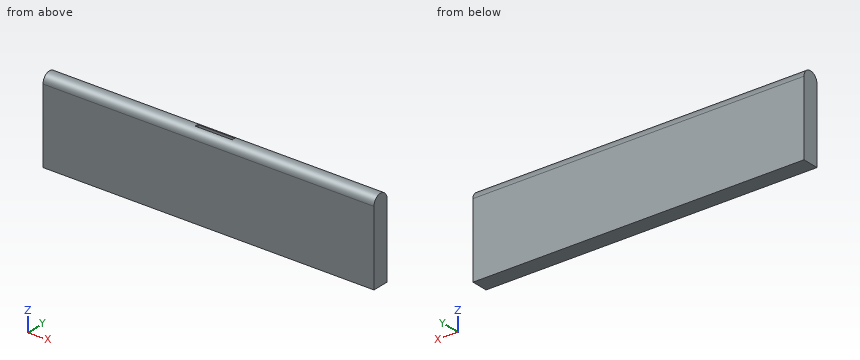
Autodesk Inventor part; units mm, degrees
ref_plane "YZ Plane" through (0, 0, 0) normal (1, 0, 0) x (0, 1, 0)
ref_plane "XZ Plane" through (0, 0, 0) normal (0, 1, 0) x (-1, 0, 0)
ref_plane "XY Plane" through (0, 0, 0) normal (0, 0, 1) x (1, 0, 0)
sketch "Sketch2" plane through (0, 0, 0) normal (0, 1, 0) x (-1, 0, 0)
  line L0 (0, 0) -> (-100, 0)
  line L1 (-100, 0) -> (-100, 25)
  line L2 (-100, 25) -> (0, 25)
  line L3 (0, 25) -> (0, 0)
  dimension "d10" = 100
  dimension "d11" = 25
extrude "Extrusion2" add sketch "Sketch2" along normal blind 5
sketch "Sketch3" plane through (0, 0, 25) normal (0, 0, 1) x (1, 0, 0)
  line L0 (0, 0) -> (100, 0) construction
  line L1 (0, 0) -> (44.4, 0) construction
  line L2 (44.4, 0) -> (44.4, 2) construction
  line L3 (44.4, 2) -> (0, 2) construction
  line L4 (0, 2) -> (0, 0) construction
  line L5 (44.4, 2) -> (55.6, 2)
  line L6 (55.6, 2) -> (55.6, 3)
  line L7 (55.6, 3) -> (44.4, 3)
  line L8 (44.4, 3) -> (44.4, 2)
  dimension "d14" = 44.4
  dimension "d15" = 2
  dimension "d16" = 11.2
  dimension "d17" = 1
extrude "Extrusion3" cut sketch "Sketch3" against normal blind 12.5
fillet "Fillet2" radius 2.5 2 edges at (50, 5, 25) (50, 0, 25)
shell "Shell1" thickness 1 removed faces 0
properties part number "RCPlaneElevator"
CAD build for the part. Positions are in the model's coordinates, mm. Coordinates: 2 decimals unless noted, no trailing zeros. Loops run counter-clockwise (first coordinate to the right, second up) from the corner with the lowest first, then second, coordinate; pieces in that order, holes last. Notation, with made-up numbers: (39.25, -30.75) - (89.25, -30.75) arc R25 cw to (89.25, -7.75) - close; hole circle Ø2 at (47.5, 56.25). An arc over 180 degrees is marked (long way). Return JSON: item names as keys, results as strings.
1. Band-saw the part on C-C (z = 19.5). Give the cut face in (x, y).
Result:
{"outline": "(0, 0) - (100, 0) - (100, 5) - (0, 5) - close; hole (1, 1) - (43.4, 1) - (43.4, 4) - (1, 4) - close; hole (44.4, 2) - (55.6, 2) - (55.6, 3) - (44.4, 3) - close; hole (56.6, 1) - (99, 1) - (99, 4) - (56.6, 4) - close"}
2. Band-saw the part on A-A (z = 2.75). Give the cut face in (x, y).
Result:
{"outline": "(0, 0) - (100, 0) - (100, 5) - (0, 5) - close; hole (1, 1) - (99, 1) - (99, 4) - (1, 4) - close"}
3. Band-saw the part on B-B (x = 87). Give the cut face in (y, z), and give its area (3 significant figures).
Result:
{"outline": "(0, 0) - (5, 0) - (5, 22.5) arc R2.5 ccw to (0, 22.5) - close; hole (1, 1) - (4, 1) - (4, 22.5) arc R1.5 ccw to (1, 22.5) - close", "area": "54.3 mm2"}
4. Drop a flat-ended pin along its axis: pin 1 (0.9 mm diameter, centred on y = 2, z = 17, fed in from -X). Give the stop position or say it passes through.
Result:
{"pin 1": "stops at x = 0"}
5. Probe L1, parallel to X at y = 1.25, z = 11.75; L2, parallel to Y at x = 70, z = 7.25; L3, parallel to X at y = 2.6, z = 14.75. List the from-to ranges inside material, lowest first. Write a range as from..to.
Result:
{"L1": "x = 0..1, 43.4..56.6, 99..100", "L2": "y = 0..1, 4..5", "L3": "x = 0..1, 43.4..44.4, 55.6..56.6, 99..100"}
